Read the model definition and answer for the solid it produces. Units are mm, in the model's axes. A direction names the side the tool comes from. Coordinates: 2 decimals unless noted, no trailing zeros. Write each loop counter-clockwise with the first axis right and the second up, starting at its lowest first coordinate (ties: lowest second). Pieces come first, ordered by that corner, then holes.
(1) Determine the mould class of faces 1 (the cylindrical face through (-2, 0, 48)), 2 (the flat face through (-3.2, 0, 0)), 3 (the flat face through (-3.3, 0.2, 12.7)) for opening direction Z: pulls with the +Z half, pulls with the -Z half, needs draft (parallel to the pull), parting line crosses it, or undercut.
(2) Which of the six approach directions +Z, -Z, +X, -X, +Y, -Y give full straight-line access (tool end or side, diameter ignored) to faces 4 (the flat face through (-2.6, -3.975, 27.4)), 5 (the flat face through (-0.5, -4.5, 48.8)), 6 (the flat face through (-2.5, 5, 49)), 7 (the cylindrical face through (-4.5, 0.1, 36.9))?
(3) The part is cut by section D-D, the plane y = 0. State how many separate pieces and enclosed holes the cut face has, and give its area (3 significant figures).
(4) The part is cut by section A-A, the plane z = 38.5. Determine the outline of the cut face in (x, y) (3 decimals), and give its area (3 significant figures).
(5) The part is cut by section C-C, the plane x = 1.5. Determine the outline of the cut face in (y, z).
(6) The part is cut by section B-B, the plane y = -6. Determine the outline of the cut face in (x, z), and give its area (3 significant figures).
(7) Given pin 1 (1.5 mm diameter, centred on x = 0.5, y = 2, fed in from -Z); pin 2 (4 mm diameter, centred on x = 0.5, y = 8, fed in from -Z); pin 3 (2 mm diameter, centred on x = -2.5, y = 0, fed in from -Z); pin 4 (0.7 mm diameter, centred on x = -3, z = 46, fed in from +Y), each flat-ended and moving along its own axis, determine where each tip first touches the part or whether it passes through.
(8) Straight lines are drawn through the part: line 1 along X through (y, z) = (-7.5, 49.8); line 2 along Y through (x, z) = (-2.25, 28); line 3 along Z through (x, y) = (-3.5, -1). For each, find the intervals that lie inside material, in ascending order.
```python
from build123d import *

# Parameters (mm, degrees)
BOSS_EXTRUDE2_DEPTH     = 51
SKETCH4_W               = 2
SKETCH4_H               = 3.5
SKETCH4_W_2             = 1.6
SKETCH4_H_2             = 2.2
SKETCH4_H_3             = 22
SKETCH4_H_4             = 0.5
SKETCH4_H_5             = 0.6
CUT_EXTRUDE1_DEPTH      = 52.487862647
CUT_EXTRUDE1_DEPTH_BACK = 52.487862647
SHELL1_DEPTH            = 23
SHELL1_START            = 48.2
SHELL1_2_DEPTH          = 2.3
SHELL1_START_2          = 23
SHELL1_3_DEPTH          = 2.2
SHELL1_START_3          = 20.5
SHELL1_4_DEPTH          = 2.5
CUT_EXTRUDE2_DEPTH      = 52.487862766
CUT_EXTRUDE2_DEPTH_BACK = 52.487862766
SKETCH11_3_W            = 2.6
SKETCH11_3_H            = 7.949874372
SKETCH11_3_H_2          = 4.92820323
BOSS_EXTRUDE3_START     = -1.206049
SKETCH13_R              = 2.5
SKETCH13_R_2            = 2
BOSS_EXTRUDE3_DEPTH     = 1.206049
SKETCH13_3_R            = 2.5
SKETCH13_3_R_2          = 2
BOSS_EXTRUDE4_DEPTH     = 1.093951
CUT_EXTRUDE3_START      = -0.2
SKETCH13_6_R            = 2.5
SKETCH13_6_R_2          = 2
CUT_EXTRUDE3_DEPTH      = 0.2
CUT_EXTRUDE4_START      = -0.2
SKETCH13_7_R            = 2.5
SKETCH13_7_R_2          = 2
CUT_EXTRUDE4_DEPTH      = 0.2
SKETCH16_W              = 0.218836676
SKETCH16_H              = 0.970663166
SKETCH16_W_2            = 0.2
SKETCH16_H_2            = 1.122183611
BOSS_EXTRUDE10_DEPTH    = 0.5


# Read off the part's stored shape, not the designer's step: Shell1
with BuildPart() as part:
    # Sketch1 → Boss-Extrude2 (new body)
    with BuildSketch(Plane.XY):
        with BuildLine():
            Line((0, 5), (0, -5))
            ThreePointArc((0, -5), (-5, 0), (0, 5))
        make_face()
    extrude(amount=BOSS_EXTRUDE2_DEPTH)

    # Sketch4 → Cut-Revolve1 (revolve, cut)
    with BuildSketch(Plane(origin=(0, 0, 0), x_dir=(1, 0, 0), z_dir=(0, 1, 0))):
        Polygon((-3, 0), (-3, -20), (-2, -20), (0, -20), (0, 0), align=None)
        with Locations((-1, -21.75)):
            Rectangle(SKETCH4_W, SKETCH4_H)
        with Locations((-2.8, -24.6)):
            Rectangle(SKETCH4_W_2, SKETCH4_H_2)
        with Locations((-1, -24.6)):
            Rectangle(SKETCH4_W, SKETCH4_H_2)
        Polygon((-2, -47.7), (-2, -25.7), (-3.6, -25.7), (-4.5, -25.7), (-4.5, -47.7), align=None)
        with Locations((-1, -36.7)):
            Rectangle(SKETCH4_W, SKETCH4_H_3)
        with Locations((-1, -47.95)):
            Rectangle(SKETCH4_W, SKETCH4_H_4)
        with Locations((-2.8, -49.3)):
            Rectangle(SKETCH4_W_2, SKETCH4_H_2)
        with Locations((-1, -49.3)):
            Rectangle(SKETCH4_W, SKETCH4_H_2)
        with Locations((-1, -50.7)):
            Rectangle(SKETCH4_W, SKETCH4_H_5)
    revolve(axis=Axis((0, 0, 0), (0, 0, 1)), mode=Mode.SUBTRACT)

    # Sketch5 → Cut-Extrude1 (cut, two sides: drawn at the far end of the back side and taken through both)
    with BuildSketch(Plane(origin=(0, 0, 0), x_dir=(1, 0, 0), z_dir=(0, 1, 0)).offset(-CUT_EXTRUDE1_DEPTH_BACK)):
        with BuildLine():
            Line((0.625, -26.325), (0.625, -47.075))
            ThreePointArc((0.625, -47.075), (0, -47.7), (-0.625, -47.075))
            Line((-0.625, -47.075), (-0.625, -26.325))
            ThreePointArc((-0.625, -26.325), (0, -25.7), (0.625, -26.325))
        make_face()
    extrude(amount=CUT_EXTRUDE1_DEPTH + CUT_EXTRUDE1_DEPTH_BACK, mode=Mode.SUBTRACT)

    # Shell1 outline → Shell1 (cut)
    with BuildSketch(Plane.XY):
        with BuildLine():
            ThreePointArc((-0.5, -3.464101615), (-3.5, 0), (-0.5, 3.464101615))
            Line((-0.5, 3.464101615), (-0.5, 4.974937186))
            ThreePointArc((-0.5, 4.974937186), (-5, 0), (-0.5, -4.974937186))
            Line((-0.5, -4.974937186), (-0.5, -3.464101615))
        make_face()
    extrude(amount=SHELL1_DEPTH, mode=Mode.SUBTRACT)

    # Shell1 2 outline → Shell1 2 (cut)
    with BuildSketch(Plane.XY.offset(SHELL1_START)):
        with BuildLine():
            Line((-0.5, -4.974937186), (-0.5, -4.06939799))
            ThreePointArc((-0.5, -4.06939799), (-4.1, 0), (-0.5, 4.06939799))
            Line((-0.5, 4.06939799), (-0.5, 4.974937186))
            ThreePointArc((-0.5, 4.974937186), (-5, 0), (-0.5, -4.974937186))
        make_face()
    extrude(amount=SHELL1_2_DEPTH, mode=Mode.SUBTRACT)

    # Shell1 3 outline → Shell1 3 (cut)
    with BuildSketch(Plane.XY.offset(SHELL1_START_2)):
        with BuildLine():
            Line((-0.5, -4.974937186), (-0.5, -4.06939799))
            ThreePointArc((-0.5, -4.06939799), (-4.1, 0), (-0.5, 4.06939799))
            Line((-0.5, 4.06939799), (-0.5, 4.974937186))
            ThreePointArc((-0.5, 4.974937186), (-5, 0), (-0.5, -4.974937186))
        make_face()
    extrude(amount=SHELL1_3_DEPTH, mode=Mode.SUBTRACT)

    # Shell1 4 outline → Shell1 4 (cut)
    with BuildSketch(Plane.XY.offset(SHELL1_START_3)):
        with BuildLine():
            Line((-0.5, -3.464101615), (-0.5, -2.449489743))
            ThreePointArc((-0.5, -2.449489743), (-2.5, 0), (-0.5, 2.449489743))
            Line((-0.5, 2.449489743), (-0.5, 3.464101615))
            ThreePointArc((-0.5, 3.464101615), (-3.5, 0), (-0.5, -3.464101615))
        make_face()
    extrude(amount=SHELL1_4_DEPTH, mode=Mode.SUBTRACT)

    # Sketch11<3> → Cut-Extrude2 (cut, two sides: drawn at the far end of the back side and taken through both)
    with BuildSketch(Plane.ZY.offset(5).offset(-CUT_EXTRUDE2_DEPTH_BACK)):
        with Locations((27.4, 0)):
            Rectangle(SKETCH11_3_W, SKETCH11_3_H)
        with Locations((34.8, 0)):
            Rectangle(SKETCH11_3_W, SKETCH11_3_H)
        with Locations((38.5, 0)):
            Rectangle(SKETCH11_3_W, SKETCH11_3_H)
        with Locations((42.2, 0)):
            Rectangle(SKETCH11_3_W, SKETCH11_3_H)
        with Locations((45.9, 0)):
            Rectangle(SKETCH11_3_W, SKETCH11_3_H)
        with Locations((2.3, 0)):
            Rectangle(SKETCH11_3_W, SKETCH11_3_H_2)
        with Locations((6.2, 0)):
            Rectangle(SKETCH11_3_W, SKETCH11_3_H_2)
        with Locations((10.1, 0)):
            Rectangle(SKETCH11_3_W, SKETCH11_3_H_2)
        with Locations((14, 0)):
            Rectangle(SKETCH11_3_W, SKETCH11_3_H_2)
        with Locations((17.9, 0)):
            Rectangle(SKETCH11_3_W, SKETCH11_3_H_2)
        with Locations((31.1, 0)):
            Rectangle(SKETCH11_3_W, SKETCH11_3_H)
    extrude(amount=CUT_EXTRUDE2_DEPTH + CUT_EXTRUDE2_DEPTH_BACK, mode=Mode.SUBTRACT)

    # Sketch13 → Boss-Extrude3 (add)
    # profile 1 of 2: a face of its own
    with BuildSketch(Plane.XY.offset(49.40604876).offset(BOSS_EXTRUDE3_START)):
        with Locations((0, 7.5)):
            Circle(SKETCH13_R)
        with Locations((0, 7.5)):
            Circle(SKETCH13_R_2, mode=Mode.SUBTRACT)
    # profile 2 of 2: a face of its own
    with BuildSketch(Plane.XY.offset(49.40604876).offset(BOSS_EXTRUDE3_START)):
        with BuildLine():
            Line((0, 4.1), (0, 5))
            ThreePointArc((0, 5), (-1.767766953, 5.732233047), (-2.5, 7.5))
            Line((-2.5, 7.5), (-2.5, 3.249615362))
            ThreePointArc((-2.5, 3.249615362), (-1.320336513, 3.881586208), (0, 4.1))
        make_face()
    extrude(amount=BOSS_EXTRUDE3_DEPTH)

    # Sketch13<3> → Boss-Extrude4 (add)
    # profile 1 of 2: a face of its own
    with BuildSketch(Plane.XY.offset(49.40604876)):
        with Locations((0, -7.5)):
            Circle(SKETCH13_3_R)
        with Locations(Location((0, -7.5, 0), (0, 0, 180))):
            Circle(SKETCH13_3_R_2, mode=Mode.SUBTRACT)
    # profile 2 of 2: a face of its own
    with BuildSketch(Plane.XY.offset(49.40604876)):
        with BuildLine():
            ThreePointArc((-2.5, -7.5), (-1.767766953, -5.732233047), (0, -5))
            Line((0, -5), (0, -4.1))
            ThreePointArc((0, -4.1), (-1.320336513, -3.881586208), (-2.5, -3.249615362))
            Line((-2.5, -3.249615362), (-2.5, -7.5))
        make_face()
    extrude(amount=BOSS_EXTRUDE4_DEPTH)

    # Sketch13<6> → Cut-Extrude3 (cut)
    # profile 1 of 2: a face of its own
    with BuildSketch(Plane.XY.offset(49.40604876).offset(CUT_EXTRUDE3_START)):
        with BuildLine():
            Line((0, 4.1), (0, 5))
            ThreePointArc((0, 5), (-1.767766953, 5.732233047), (-2.5, 7.5))
            Line((-2.5, 7.5), (-2.5, 3.249615362))
            ThreePointArc((-2.5, 3.249615362), (-1.320336513, 3.881586208), (0, 4.1))
        make_face()
    # profile 2 of 2: a face of its own
    with BuildSketch(Plane.XY.offset(49.40604876).offset(CUT_EXTRUDE3_START)):
        with Locations((0, 7.5)):
            Circle(SKETCH13_6_R)
        with Locations((0, 7.5)):
            Circle(SKETCH13_6_R_2, mode=Mode.SUBTRACT)
    extrude(amount=CUT_EXTRUDE3_DEPTH, mode=Mode.SUBTRACT)

    # Sketch13<7> → Cut-Extrude4 (cut)
    # profile 1 of 2: a face of its own
    with BuildSketch(Plane.XY.offset(49.40604876).offset(CUT_EXTRUDE4_START)):
        with Locations((0, -7.5)):
            Circle(SKETCH13_7_R)
        with Locations(Location((0, -7.5, 0), (0, 0, 180))):
            Circle(SKETCH13_7_R_2, mode=Mode.SUBTRACT)
    # profile 2 of 2: a face of its own
    with BuildSketch(Plane.XY.offset(49.40604876).offset(CUT_EXTRUDE4_START)):
        with BuildLine():
            ThreePointArc((-2.5, -7.5), (-1.767766953, -5.732233047), (0, -5))
            Line((0, -5), (0, -4.1))
            ThreePointArc((0, -4.1), (-1.320336513, -3.881586208), (-2.5, -3.249615362))
            Line((-2.5, -3.249615362), (-2.5, -7.5))
        make_face()
    extrude(amount=CUT_EXTRUDE4_DEPTH, mode=Mode.SUBTRACT)

    # Sketch16 → Boss-Extrude10 (add)
    with BuildSketch(Plane(origin=(0, 0, 0), x_dir=(0, 0, -1), z_dir=(1, 0, 0))):
        with Locations((-49.315467098, -4.514668417)):
            Rectangle(SKETCH16_W, SKETCH16_H)
        with Locations((-49.30604876, 4.509747926)):
            Rectangle(SKETCH16_W_2, SKETCH16_H_2)
    extrude(amount=-BOSS_EXTRUDE10_DEPTH)


solid = part.part
```
Computed:
1. face 1: needs draft
1. face 2: pulls with the -Z half
1. face 3: undercut
2. face 4: +X, -X
2. face 5: -X, -Y
2. face 6: -X, +Y
2. face 7: +X
3. separate pieces: 12
3. enclosed holes: 0
3. area: 15.6 mm2
4. outline: (-3.033, -3.975) arc R5 ccw to (-0.625, -4.961) - (-0.625, -4.456) arc R4.5 cw to (-2.109, -3.975) - close; (-3.033, 3.975) - (-2.109, 3.975) arc R4.5 cw to (-0.625, 4.456) - (-0.625, 4.961) arc R5 ccw to start
4. area: 2.12 mm2
5. outline: (-9.5, 49.41) - (-8.82, 49.41) - (-8.82, 50.5) - (-9.5, 50.5) - close; (-6.18, 49.41) - (-5.5, 49.41) - (-5.5, 50.5) - (-6.18, 50.5) - close; (5.5, 48.2) - (6.18, 48.2) - (6.18, 49.21) - (5.5, 49.21) - close; (8.82, 48.2) - (9.5, 48.2) - (9.5, 49.21) - (8.82, 49.21) - close
6. outline: (-2.5, 49.41) - (-1.32, 49.41) - (-1.32, 50.5) - (-2.5, 50.5) - close; (1.32, 49.41) - (2, 49.41) - (2, 50.5) - (1.32, 50.5) - close
6. area: 2.03 mm2
7. pin 1: stops at z = 20
7. pin 2: stops at z = 48.2
7. pin 3: stops at z = 0
7. pin 4: stops at y = 4.24
8. line 1: x = -2.5 to -2, 2 to 2.5
8. line 2: y = -4.47 to -3.97, 3.97 to 4.47
8. line 3: z = 23 to 25.7, 47.7 to 51
